Input: part model. Units: mm. Frame: model coordinates. A direction names the side the tool comes from. Give positions to 0.01 mm unless a question says otherwise; leave off trailing zeros. Order: outer loops, then holes, each group sorted by start corner. A loop starts at its lowest first (then second) coordinate and runs counter-clockwise, first axis right, second up. Notation, with made-up numbers: M 72,59.5 L 116,59.5 A33 cw 116,87.5 Z; hole C -13.5,82.5 d9. An arc over 180 degrees is marked long. Use a Markdown table: item, result.
from build123d import *

# Parameters (mm, degrees)
F0_W     = 57.15
F0_H     = 44.45
F1_DEPTH = 25.4
F3_DEPTH = 12.7
F4_DEPTH = 25.4


with BuildPart() as f1:
    # F0 (on Front) → F1 (new body)
    with BuildSketch(Plane.XZ):
        with Locations((-30.2558824187, 38.2586528428)):
            Rectangle(F0_W, F0_H)
    extrude(amount=F1_DEPTH)

    # F2 (on face) → F3 (cut)
    with BuildSketch(Plane.XZ.offset(25.4)):
        with BuildLine():
            ThreePointArc((-17.3336963264, 43.7719967953), (-23.7576790398, 54.9273203296), (-36.6304001601, 54.9703088903))
            Line((-36.6304001601, 54.9703088903), (-23.8323291944, 32.5736847003))
            ThreePointArc((-23.8323291944, 32.5736847003), (-19.0760411429, 37.2983111579), (-17.3336963264, 43.7719967953))
        make_face()
        with BuildLine():
            Line((-23.8323291944, 32.5736847003), (-36.6304001601, 54.9703088903))
            ThreePointArc((-36.6304001601, 54.9703088903), (-41.4296767723, 37.3729613124), (-23.8323291944, 32.5736847003))
        make_face()
        with BuildLine():
            Line((-1.6808824187, 60.4836528428), (-39.7808824187, 60.4836528428))
            Line((-39.7808824187, 60.4836528428), (-36.6304001601, 54.9703088903))
            ThreePointArc((-36.6304001601, 54.9703088903), (-23.7576790398, 54.9273203296), (-17.3336963264, 43.7719967953))
            ThreePointArc((-17.3336963264, 43.7719967953), (-19.0760411429, 37.2983111579), (-23.8323291944, 32.5736847003))
            Line((-23.8323291944, 32.5736847003), (-14.3808824187, 16.0336528428))
            Line((-14.3808824187, 16.0336528428), (-1.6808824187, 16.0336528428))
            Line((-1.6808824187, 16.0336528428), (-1.6808824187, 60.4836528428))
        make_face()
    extrude(amount=-F3_DEPTH, mode=Mode.SUBTRACT)

    # F2 (on face) → F4 (cut)
    with BuildSketch(Plane.XZ.offset(25.4)):
        with BuildLine():
            ThreePointArc((-17.3336963264, 43.7719967953), (-23.7576790398, 54.9273203296), (-36.6304001601, 54.9703088903))
            Line((-36.6304001601, 54.9703088903), (-23.8323291944, 32.5736847003))
            ThreePointArc((-23.8323291944, 32.5736847003), (-19.0760411429, 37.2983111579), (-17.3336963264, 43.7719967953))
        make_face()
        with BuildLine():
            Line((-23.8323291944, 32.5736847003), (-36.6304001601, 54.9703088903))
            ThreePointArc((-36.6304001601, 54.9703088903), (-41.4296767723, 37.3729613124), (-23.8323291944, 32.5736847003))
        make_face()
    extrude(amount=-F4_DEPTH, mode=Mode.SUBTRACT)


solid = f1.part
1) Cut plane A-A on y = -5. Return loops of the section in (x, z).
Response values:
| item | result |
|---|---|
| outline | M -58.83,16.03 L -1.68,16.03 L -1.68,60.48 L -58.83,60.48 Z; hole C -30.23,43.77 d25.8 |
2) Cut plane D-D on y = -18. Return loops of the section in (x, z).
Response values:
| item | result |
|---|---|
| outline | M -58.83,16.03 L -14.38,16.03 L -23.83,32.57 A12.9 cw -36.63,54.97 L -39.78,60.48 L -58.83,60.48 Z |
3) Material intervals for line 1 (Z direction, x = -19, y = -12); line 2 (X direction, y = -1.5, z = 49); line 3 (Y direction, x = -7, z = 49.5), sorted ascending. Write a range as from..to.
Response values:
| item | result |
|---|---|
| line 1 | z = 16.03..37.43, 50.11..60.48 |
| line 2 | x = -58.83..-42.02, -18.44..-1.68 |
| line 3 | y = -12.7..0 |
4) Cut plane B-B on x = -27.5. Return loops of the section in (y, z).
Response values:
| item | result |
|---|---|
| outline | M -25.4,16.03 L 0,16.03 L 0,31.17 L -25.4,31.17 Z; M -12.7,56.38 L 0,56.38 L 0,60.48 L -12.7,60.48 Z |
5) Reachability of faces 1 (the face through (-38.23, -19.14, 57.77)), 2 (the face through (-37, -10, 60.484)) from +Z, -Z, +X, -X, +Y, -Y: full face, straight path, thin tool, end or side. Return the list, or none.
Response values:
| item | result |
|---|---|
| face 1 | +Z, +X, -Y |
| face 2 | +Z, +X, -X, +Y, -Y |
6) First-contact query: pin 1 Ø4 at (x, y) = (-16.5, -17.5) entering from +Z. Flat tip, straight axial feed; report the tip coordinate or a pass-through.
Response values:
| item | result |
|---|---|
| pin 1 | stops at z = 23.24 |
7) Cut plane C-C on z = 45. Return loops of the section in (x, y).
Response values:
| item | result |
|---|---|
| outline | M -58.83,-25.4 L -43.07,-25.4 L -43.07,0 L -58.83,0 Z; M -17.39,-12.7 L -1.68,-12.7 L -1.68,0 L -17.39,0 Z |
